```python
from build123d import *

# Parameters (mm, degrees)
F0_W     = 70
F0_H     = 50
F1_DEPTH = 150
F2_T     = -2.5
F4_DEPTH = 2


with BuildPart() as f1:
    # F0 (on Right) → F1 (new body)
    with BuildSketch(Plane.YZ):
        with Locations((35, 25)):
            Rectangle(F0_W, F0_H)
    extrude(amount=F1_DEPTH)

    # F2
    f2_openings = [f1.faces().sort_by_distance(p)[0] for p in [
        (75, 35, 0),
    ]]
    offset(amount=F2_T, openings=f2_openings)

    # F3 (on Front) → F4 (join)
    with BuildSketch(Plane.XZ):
        with BuildLine():
            Line((57.11453, 36.209103), (47.46139, 36.209103))
            ThreePointArc((47.46139, 36.209103), (45.909707, 34.307581), (47.600284, 32.528408))
            Line((47.600284, 32.528408), (49.579524, 32.389514))
            Line((49.579524, 32.389514), (49.579524, 27.944904))
            ThreePointArc((49.579524, 27.944904), (50.38126, 27.095251), (51.50668, 26.782002))
            ThreePointArc((51.50668, 26.782002), (52.632099, 27.095251), (53.433836, 27.944904))
            Line((53.433836, 27.944904), (53.433836, 29.116847))
            Line((53.433836, 29.116847), (53.433836, 32.389514))
            Line((53.433836, 32.389514), (55.413075, 32.389514))
            Line((55.413075, 32.389514), (55.413075, 27.944904))
            ThreePointArc((55.413075, 27.944904), (57.374954, 26.432392), (59.336834, 27.944904))
            Line((59.336834, 27.944904), (59.336834, 33.917353))
            ThreePointArc((59.336834, 33.917353), (58.710678, 35.533527), (57.11453, 36.209103))
        make_face()
        with BuildLine():
            ThreePointArc((53.433836, 27.944904), (52.632099, 27.095251), (51.50668, 26.782002))
            Line((51.50668, 26.782002), (51.50668, 25.973246))
            Line((51.50668, 25.973246), (46.945356, 25.973246))
            ThreePointArc((46.945356, 25.973246), (45.1954, 24.223289), (46.945356, 22.473333))
            Line((46.945356, 22.473333), (51.845234, 22.473333))
            Line((51.845234, 22.473333), (51.845234, 19.279664))
            Line((51.845234, 19.279664), (49.132802, 19.279664))
            ThreePointArc((49.132802, 19.279664), (47.470343, 17.617206), (49.132802, 15.954748))
            Line((49.132802, 15.954748), (51.232748, 15.954748))
            Line((51.232748, 15.954748), (49.132802, 13.548559))
            ThreePointArc((49.132802, 13.548559), (49.262718, 11.31813), (51.495243, 11.404863))
            Line((51.495243, 11.404863), (53.551439, 14.24854))
            Line((53.551439, 14.24854), (55.388894, 11.404863))
            ThreePointArc((55.388894, 11.404863), (57.530578, 10.996438), (57.838831, 13.154818))
            Line((57.838831, 13.154818), (55.80093, 15.74391))
            Line((55.80093, 15.74391), (58.145076, 15.74391))
            Line((58.145076, 15.74391), (73.538758, 15.648505))
            Line((73.538758, 15.648505), (73.538758, 18.361211))
            Line((73.538758, 18.361211), (70.587255, 18.361211))
            Line((70.587255, 18.361211), (70.587255, 19.2293))
            Line((70.587255, 19.2293), (73.538758, 19.2293))
            Line((73.538758, 19.2293), (73.538758, 21.79884))
            Line((73.538758, 21.79884), (67.63576, 21.79884))
            Line((67.63576, 21.79884), (67.63576, 17.66674))
            Line((67.63576, 17.66674), (64.927325, 17.66674))
            Line((64.927325, 17.66674), (64.927325, 18.916788))
            Line((64.927325, 18.916788), (67.149632, 18.916788))
            Line((67.149632, 18.916788), (67.149632, 26.104558))
            Line((67.149632, 26.104558), (64.510643, 26.104558))
            Line((64.510643, 26.104558), (64.510643, 24.472551))
            Line((64.510643, 24.472551), (63.399486, 24.472551))
            Line((63.399486, 24.472551), (63.399486, 26.104558))
            Line((63.399486, 26.104558), (54.681171, 26.104558))
            Line((54.681171, 26.104558), (54.681171, 27.944904))
            ThreePointArc((54.681171, 27.944904), (54.310984, 28.800663), (53.433836, 29.116847))
            Line((53.433836, 29.116847), (53.433836, 27.944904))
        make_face()
        with BuildLine():
            Line((55.563889, 19.367162), (55.563889, 22.429585))
            Line((55.563889, 22.429585), (60.682509, 22.429585))
            Line((60.682509, 22.429585), (60.682509, 19.017169))
            Line((60.682509, 19.017169), (62.694959, 19.017169))
            Line((62.694959, 19.017169), (62.694959, 17.8797))
            Line((62.694959, 17.8797), (59.413794, 17.8797))
            ThreePointArc((59.413794, 17.8797), (59.113771, 18.903701), (58.145076, 19.351165))
            Line((58.145076, 19.351165), (55.563889, 19.367162))
        make_face(mode=Mode.SUBTRACT)
        Polygon((62.694959, 20.460883), (62.694959, 21.904599), (64.663664, 21.948347), (64.663664, 20.460883), align=None, mode=Mode.SUBTRACT)
        Polygon((76.495692, 21.79884), (74.030101, 21.79884), (74.030101, 15.532267), (76.495692, 15.532267), (76.495692, 16.965751), (78.674585, 16.965751), (78.674585, 19.832715), (76.495692, 19.832715), align=None)
        with BuildLine():
            Line((91.996334, 12.50622), (91.996334, 21.270147))
            Line((91.996334, 21.270147), (81.880391, 21.270147))
            Line((81.880391, 21.270147), (81.880391, 12.74765))
            Line((81.880391, 12.74765), (85.50185, 12.74765))
            Line((85.50185, 12.74765), (85.50185, 11.347353))
            Line((85.50185, 11.347353), (81.180245, 11.347353))
            Line((81.180245, 11.347353), (81.180245, 9.633197))
            Line((81.180245, 9.633197), (81.180245, 9.335577))
            Line((81.180245, 9.335577), (85.081376, 9.335577))
            ThreePointArc((85.081376, 9.335577), (76.634992, 4.361003), (70.154078, 11.715291))
            Line((70.154078, 11.715291), (68.28817, 11.715291))
            ThreePointArc((68.28817, 11.715291), (71.119618, 4.873442), (78.023359, 2.196435))
            ThreePointArc((78.023359, 2.196435), (83.870671, 4.472691), (87.590158, 9.526185))
            Line((87.590158, 9.526185), (90.47015, 9.526185))
            Line((90.47015, 9.526185), (90.47015, 5.510417))
            Line((90.47015, 5.510417), (89.181907, 5.510417))
            Line((89.181907, 5.510417), (89.181907, 3.806551))
            Line((89.181907, 3.806551), (90.68878, 3.806551))
            ThreePointArc((90.68878, 3.806551), (91.62855, 4.383871), (91.996334, 5.423679))
            Line((91.996334, 5.423679), (91.996334, 11.00935))
            Line((91.996334, 11.00935), (87.771297, 11.00935))
            Line((87.771297, 11.00935), (87.771297, 12.50622))
            Line((87.771297, 12.50622), (91.996334, 12.50622))
        make_face()
        with BuildLine():
            ThreePointArc((86.42818, 18.893627), (86.959373, 19.572715), (87.490566, 18.893627))
            Line((87.490566, 18.893627), (87.490566, 17.541504))
            Line((87.490566, 17.541504), (88.762209, 17.541504))
            ThreePointArc((88.762209, 17.541504), (89.172675, 17.131037), (88.762209, 16.720571))
            Line((88.762209, 16.720571), (87.683722, 16.720571))
            Line((87.683722, 16.720571), (88.617332, 15.497221))
            ThreePointArc((88.617332, 15.497221), (88.694215, 15.11667), (88.442416, 14.821159))
            ThreePointArc((88.442416, 14.821159), (88.264398, 14.783906), (88.086381, 14.821159))
            Line((88.086381, 14.821159), (87.764211, 14.821159))
            Line((87.764211, 14.821159), (86.186729, 14.821159))
            Line((86.186729, 14.821159), (85.832366, 14.821159))
            ThreePointArc((85.832366, 14.821159), (85.654348, 14.783906), (85.476331, 14.821159))
            ThreePointArc((85.476331, 14.821159), (85.224532, 15.11667), (85.301414, 15.497221))
            Line((85.301414, 15.497221), (86.235024, 16.720571))
            Line((86.235024, 16.720571), (85.156538, 16.720571))
            ThreePointArc((85.156538, 16.720571), (84.746071, 17.131037), (85.156538, 17.541504))
            Line((85.156538, 17.541504), (86.42818, 17.541504))
            Line((86.42818, 17.541504), (86.42818, 18.893627))
        make_face(mode=Mode.SUBTRACT)
        with BuildLine():
            Line((106.654562, 20.205654), (95.455378, 20.205654))
            Line((95.455378, 20.205654), (95.455378, 18.35208))
            Line((95.455378, 18.35208), (101.575367, 18.35208))
            Line((101.575367, 18.35208), (103.034772, 18.35208))
            Line((103.034772, 18.35208), (102.845654, 17.135097))
            Line((102.845654, 17.135097), (101.776361, 15.61341))
            Line((101.776361, 15.61341), (100.624815, 14.338483))
            Line((100.624815, 14.338483), (100.624815, 12.600102))
            Line((100.624815, 12.600102), (93.343966, 12.600102))
            Line((93.343966, 12.600102), (93.343966, 10.864255))
            Line((93.343966, 10.864255), (100.416891, 10.864255))
            Line((100.416891, 10.864255), (100.416891, 5.193939))
            ThreePointArc((100.416891, 5.193939), (100.047414, 4.480832), (99.251762, 4.371406))
            Line((99.251762, 4.371406), (99.251762, 2.890847))
            ThreePointArc((99.251762, 2.890847), (100.685052, 3.105352), (101.390347, 4.371406))
            Line((101.390347, 4.371406), (101.390347, 10.864255))
            Line((101.390347, 10.864255), (107.559353, 10.864255))
            Line((107.559353, 10.864255), (107.559353, 12.103219))
            Line((107.559353, 12.103219), (102.212884, 12.103219))
            Line((102.212884, 12.103219), (102.212884, 13.337018))
            ThreePointArc((102.212884, 13.337018), (104.800372, 16.534238), (106.654562, 20.205654))
        make_face()
        with BuildLine():
            Line((87.764211, 14.821159), (88.086381, 14.821159))
            ThreePointArc((88.086381, 14.821159), (87.917839, 14.950376), (87.828599, 15.143093))
            Line((87.828599, 15.143093), (86.959373, 16.527411))
            Line((86.959373, 16.527411), (86.090147, 15.143093))
            ThreePointArc((86.090147, 15.143093), (86.000907, 14.950376), (85.832366, 14.821159))
            Line((85.832366, 14.821159), (86.186729, 14.821159))
            Line((86.186729, 14.821159), (87.764211, 14.821159))
        make_face()
    extrude(amount=F4_DEPTH)


solid = f1.part
```
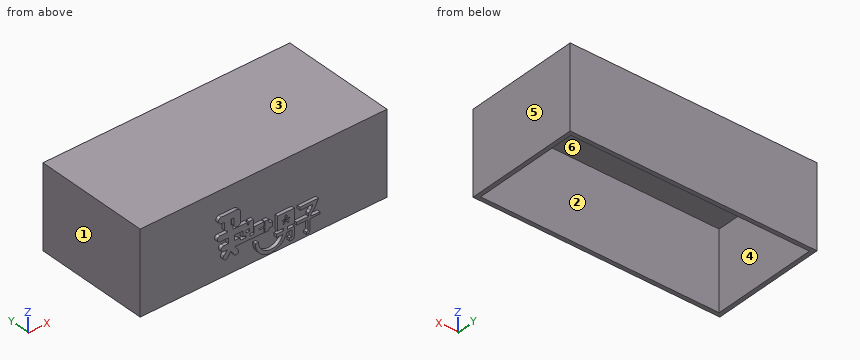
Could you check a few things on this model? Use its own coordinates, in mm. Face numbers are marked on the shaded views. A direction names the side the tool comes from. Round coordinates to 2 decimals unless told otherwise and drop trailing zeros. Loops run counter-clockwise (first coordinate to the right, second up) from the corner with the lowest first, then second, coordinate; pieces in that order, holes last. Notation, with made-up numbers: (48.25, 84) - (96.25, 84) arc R20 ccw to (96.25, 123) - close; hole circle Ø7 at (-32, 84.25). An arc over 180 degrees is marked (long way). Answer in a Markdown table with one row per item. Add a question column.
(1) If we mould it in two halves opening along X, with no side actions, what happens to the marked faces 3, 4, 5 and 6? For each: pulls with the +X half, pulls with the -X half, needs draft (parallel to the pull), parting line crosses it, or undercut.
(2) If we section it at A-A (z = 40): Please give me the cut outline in (x, y), plus the area to 4 significant figures.
(3) I need wall thicknesses on line 1 along X through (y, z) = (33.5, 40); line 2 along Y through (x, z) = (47, 33); line 3 along Y through (x, z) = (99, 37.5). Which ranges of each line are inside material? Lowest first, please.
(4) I'm going to push flat-ended pins straight in: pin 1 (0.7 mm diameter, centred on y = -1.5, z = 21, fed in from +X); pin 2 (1.6 mm diameter, centred on x = 66, y = -1.5, fed in from +Z); pin 3 (1.6 mm diameter, centred on x = 95, y = -1, fed in from -Z). Where does each tip first touch, or does it pass through?
(5) For the marked faces 1 and 2, which set-ups out of +Z, -Z, +X, -X, +Y, -Y let a thin tool reach every point of the face, with its end or its side?
(6) If we section it at C-C (y = 25): Please give me the cut outline in (x, z).
(7) If we section it at D-D (x = 97.5): Please give me the cut outline in (y, z), plus the area to 3 significant figures.
(8) If we section it at B-B (x = 11.5): Please give me the cut outline in (y, z).
Model answer:
| question | item | result |
|---|---|---|
| 1 | face 3 | needs draft |
| 1 | face 4 | undercut |
| 1 | face 5 | pulls with the +X half |
| 1 | face 6 | undercut |
| 2 | outline | (0, 0) - (150, 0) - (150, 70) - (0, 70) - close; hole (2.5, 2.5) - (147.5, 2.5) - (147.5, 67.5) - (2.5, 67.5) - close |
| 2 | area | 1,075 mm² |
| 3 | line 1 | x = 0 to 2.5, 147.5 to 150 |
| 3 | line 2 | y = -2 to 2.5, 67.5 to 70 |
| 3 | line 3 | y = 0 to 2.5, 67.5 to 70 |
| 4 | pin 1 | stops at x = 92 |
| 4 | pin 2 | stops at z = 26.1 |
| 4 | pin 3 | stops at z = 10.86 |
| 5 | face 1 | +Z, -Z, -X, +Y, -Y |
| 5 | face 2 | -Z |
| 6 | outline | (0, 0) - (2.5, 0) - (2.5, 47.5) - (147.5, 47.5) - (147.5, 0) - (150, 0) - (150, 50) - (0, 50) - close |
| 7 | outline | (-2, 10.86) - (0, 10.86) - (0, 0) - (2.5, 0) - (2.5, 47.5) - (67.5, 47.5) - (67.5, 0) - (70, 0) - (70, 50) - (0, 50) - (0, 20.21) - (-2, 20.21) - (-2, 18.35) - (0, 18.35) - (0, 12.6) - (-2, 12.6) - close |
| 7 | area | 420 mm² |
| 8 | outline | (0, 0) - (2.5, 0) - (2.5, 47.5) - (67.5, 47.5) - (67.5, 0) - (70, 0) - (70, 50) - (0, 50) - close |
